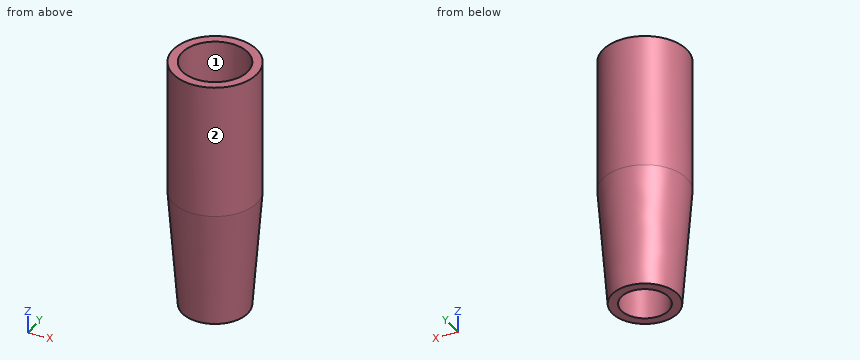
```python
from build123d import *

# Parameters (mm, degrees)
CYLINDER001_R     = 1.8
CYLINDER001_DEPTH = 7.4
CYLINDER_R        = 2.3
CYLINDER_DEPTH    = 7.4


with BuildPart() as cone001:
    # Cone001 → Cone001 (revolve)
    with BuildSketch(Plane(origin=(0, 0, -6.5), x_dir=(1, 0, 0), z_dir=(0, -1, 0))):
        Polygon((0, 0), (1.3, 0), (1.8, 6.5), (0, 6.5), align=None)
    revolve(axis=Axis((0, 0, -6.5), (0, 0, 1)))


with BuildPart() as inner_fusion:
    # Cylinder001 → Cylinder001 (new body)
    with BuildSketch(Plane.XY):
        Circle(CYLINDER001_R)
    extrude(amount=CYLINDER001_DEPTH)

    # Fusion001: union Cone001
    add(cone001.part)


with BuildPart() as cone:
    # Cone → Cone (revolve)
    with BuildSketch(Plane(origin=(0, 0, -6.5), x_dir=(1, 0, 0), z_dir=(0, -1, 0))):
        Polygon((0, 0), (1.8, 0), (2.3, 6.5), (0, 6.5), align=None)
    revolve(axis=Axis((0, 0, -6.5), (0, 0, 1)))


with BuildPart() as obj1:
    # Cylinder → Cylinder (new body)
    with BuildSketch(Plane.XY):
        Circle(CYLINDER_R)
    extrude(amount=CYLINDER_DEPTH)

    # Fusion: union Cone
    add(cone.part)

    # Cut: cut inner fusion
    add(inner_fusion.part, mode=Mode.SUBTRACT)


solid = obj1.part
```
Geometry: final body of the model. Coordinates: model frame, mm. Face numbers are marked on the shaded views. Give positions to 0.01 mm unless a question says otherwise; leave off trailing zeros. Write each loop counter-clockwise with the first axis right and the second up, starting at its lowest first coordinate (ties: lowest second). Pieces come first, ordered by that corner, then holes.
1. Pin query (flat end, axial travel): P1, Ø1.5, axis at x = 1, z = -1.5, coming from the +Y side; P2, Ø1, axis at y = -1, z = 0.5, coming from the -X side (3 decimals). Return the tip coordinate at first contact, or that it passes through.
2. Section query C-C, the plane z = 0.25. Return loops of the section in (x, y), then the cut area to 3 significant figures.
3. Line query: probe 1 along Y at (x, z) = (0, 5.75); probe 2 along Y at (x, z) = (-1.25, 1); probe 3 along X at (y, z) = (0.05, -1). Output: solid intervals per line, ascending.
4. Draft query along X for the marked faces 1 and 2. Return one class per face: released by +X, released by -X, zero draft, split by the parting line, or undercut.
5. Section query A-A, the plane x = 0. Return loops of the section in (y, z).
Computed:
1. P1: stops at y = 2.19
1. P2: stops at x = -2.245
2. outline: circle Ø4.6 at (0, 0); hole circle Ø3.6 at (0, 0)
2. area: 6.44 mm2
3. probe 1: y = -2.3 to -1.8, 1.8 to 2.3
3. probe 2: y = -1.93 to -1.3, 1.3 to 1.93
3. probe 3: x = -2.22 to -1.72, 1.72 to 2.22
4. face 1: undercut
4. face 2: split by the parting line
5. outline: (-2.3, 0) - (-1.8, -6.5) - (-1.3, -6.5) - (-1.8, 0) - (-1.8, 7.4) - (-2.3, 7.4) - close; (1.3, -6.5) - (1.8, -6.5) - (2.3, 0) - (2.3, 7.4) - (1.8, 7.4) - (1.8, 0) - close
